Here's the drawing with two shaded views (mm, measured from the low corner). I have some questions. A direction names the side the tool comes from. Round coordinates to 2 decimals unless told otherwise and drop trailing zeros. Order: outer loops, then holes, each group sorted by start corner. A loop starts at its lowest first (then second) coordinate and runs counter-clockwise, first axis right, second up. Notation, with made-up numbers: (-22, 76.5) - (10, 76.5) arc R14 ccw to (10, 89.5) - close; hole circle Ø3 at (22, 14.5). An arc over 180 degrees is marked (long way). One line per item, written item: value.
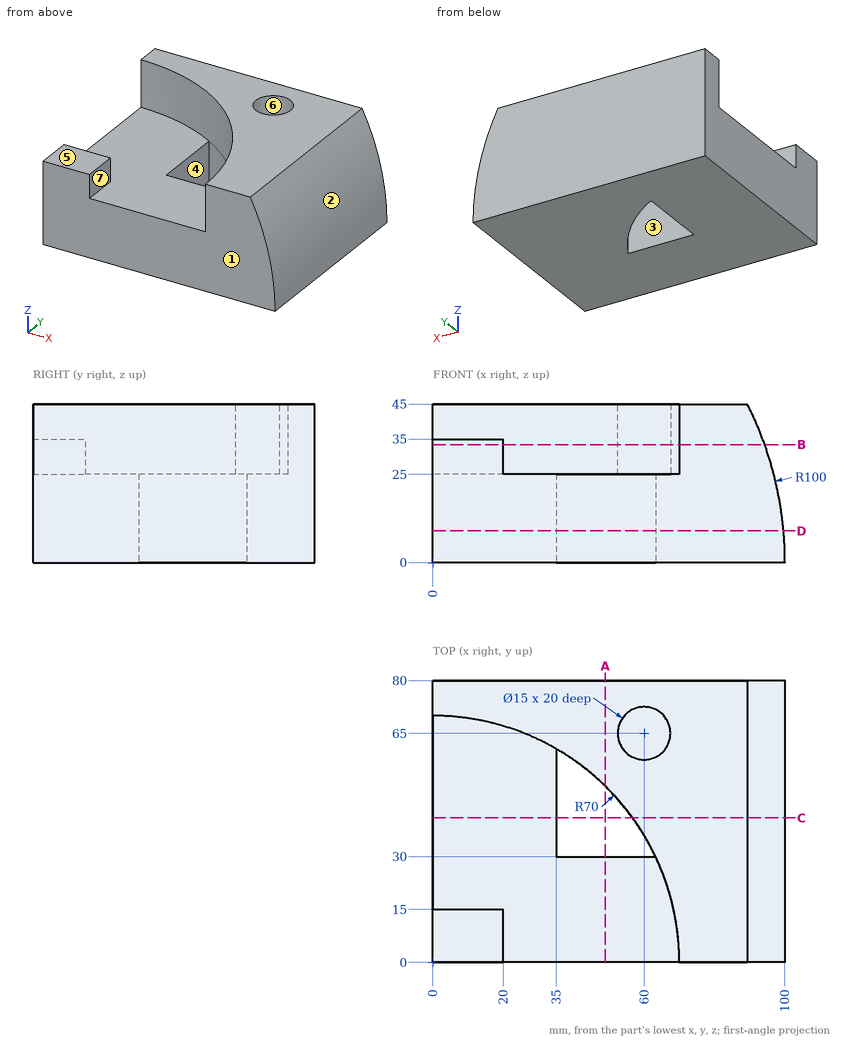
Q1. If we section it at C-C, the plane y = 41: Please give me the cut outline in (x, z), then the cut area to 4 significant figures.
Results list:
outline: (0, 0) - (35, 0) - (35, 25) - (0, 25) - close; (56.74, 0) - (100, 0) arc R100 ccw to (89.3, 45) - (56.74, 45) - close
area: 2,665 mm²
Q2. Which directions (+Z, -Z, +X, -X, +Y, -Y) give clear straight access to the entire face, cutting with the end or side of a thin tool? Please do the marked faces 4, 5, 6 and 7.
Results list:
face 4: +Z, -Z
face 5: +Z, -X, -Y
face 6: +Z
face 7: +Z, -Y
Q3. If we section it at B-B, the plane z = 33.5: Please give me the cut outline in (x, y), then the cut area to 3 significant figures.
Results list:
outline: (0, 0) - (20, 0) - (20, 15) - (0, 15) - close; (0, 70) arc R70 cw to (70, 0) - (94.22, 0) - (94.22, 80) - (0, 80) - close; hole circle Ø15 at (60, 65)
area: 3,810 mm²
Q4. If we section it at A-A, the plane x = 49: Please give me the cut outline in (y, z), then the cut area to 3 significant figures.
Results list:
outline: (0, 0) - (30, 0) - (30, 25) - (0, 25) - close; (49.99, 0) - (80, 0) - (80, 45) - (49.99, 45) - close
area: 2,100 mm²
Q5. We'd pull the mould along Y, two halves only. Please class the marked faces 1, 2 and 3: released by +Y, released by -Y, zero draft, split by the parting line, or undercut.
Results list:
face 1: released by -Y
face 2: zero draft
face 3: undercut
Q6. If we section it at D-D, the plane z = 9: Please give me the cut outline in (x, y).
Results list:
outline: (0, 0) - (99.59, 0) - (99.59, 80) - (0, 80) - close; hole (35, 30) - (63.25, 30) arc R70 ccw to (35, 60.62) - close
Q7. If I drill on line 1 along Y through (x, z) = (17.5, 30); line 2 along Y through (x, z) = (60, 39); line 3 along Z through (x, y) = (7.5, 31), over which ranges is the centre line in solid material (lowest first)?
Results list:
line 1: 0 to 15, 67.78 to 80
line 2: 36.06 to 57.5, 72.5 to 80
line 3: 0 to 25
Q8. Will these pins go through, and if not, where does the flat tip stop? pin 1 (8 mm diameter, centred on x = 27, y = 8.5, fed in from +Z); pin 2 (10 mm diameter, centred on y = 59, z = 36, fed in from -X); pin 3 (1.5 mm diameter, centred on y = 58.5, z = 28.5, fed in from +X).
Results list:
pin 1: z = 25
pin 2: x = 28.35
pin 3: x = 96.07
